Can you work these out from the model? Positions are in its coordinate system, mm. Coordinates: 2 decimals unless noted, no trailing zeros. Loops run counter-clockwise (first coordinate to the right, second up) from the corner with the lowest first, then second, coordinate; pieces in that order, holes last. Notation, with made-up numbers: M 55.5,26 L 65.5,26 A13 ccw 65.5,51 Z; hole C 2.25,-30.5 d7. An arc over 180 degrees is marked long. Answer as a JSON object with one key per item and string values. Group by question number.
Item 1: Suppose I cut it at C-C (y = -11). Write out the boundary of the cut face in (x, z).
Item 2: I'm going to push a flat-ended pin straight in: pin 1 Ø2 at (y, z) = (-6, 1) entering from -X. Where does the tip first touch, or does it pass through?
Item 3: Suppose I cut it at A-A (z = 0). Write out the boundary of the cut face in (x, y), then the cut area to 3 significant figures.
Item 4: Suppose I cut it at B-B (y = 2.75). Write out the boundary of the cut face in (x, z), then the cut area to 3 significant figures.
Item 5: If I drill on line 1 (X direction, y = -0.25, z = 0); line 2 (X direction, y = -11.25, z = 0.75); line 3 (Y direction, x = -1.25, z = -3), over which ranges is the centre line in solid material (lowest first)?
Item 6: We'd pull the mould along X, two halves only. Please class faces 1 (the flat face through (2, 3.781, 0)), 2 (the cylindrical face through (-0.1, -5.3, -2.5)), 3 (the flat face through (0.37, 3.02, 0.06)), 4 (the flat face through (-0.38, 3.04, 0.06)): +X half, -X half, draft (parallel to the pull), parting line (faces both ways), or undercut.
```python
from build123d import *

# Parameters (mm, degrees)
EXTRUDE1_DEPTH = 5


with BuildPart() as part:
    # Sketch1 → Revolve1 (revolve)
    with BuildSketch(Plane.XY, mode=Mode.PRIVATE) as revolve1_sk:
        Polygon((0, 3.780981067), (4.5, 3.780981067), (2.5, 1.780981067), (2.5, -12.219018933), (0, -12.219018933), align=None)
    revolve(revolve1_sk.sketch.rotate(Axis((0, 84.539156627, 0), (0, -1, 0)), 90), axis=Axis((0, 84.539156627, 0), (0, -1, 0)))

    # Sketch2 → Extrude1 (cut, symmetric)
    with BuildSketch(Plane.XY):
        Polygon((-0.75, 3.780981067), (0, 2.280981067), (0.75, 3.780981067), align=None)
    extrude(amount=EXTRUDE1_DEPTH, both=True, mode=Mode.SUBTRACT)


solid = part.part
```
From the geometry:
{
 "1": {"outline": "C 0,0 d5"},
 "2": {"pin 1": "x = -2.5"},
 "3": {"outline": "M -4.5,3.78 L -2.5,1.78 L -2.5,-12.22 L 2.5,-12.22 L 2.5,1.78 L 4.5,3.78 L 0.75,3.78 L 0,2.28 L -0.75,3.78 Z", "area": "82.9 mm2"},
 "4": {"outline": "M -0.23,-3.46 L -0.23,3.46 A3.47 ccw Z; M 0.23,-3.46 A3.47 ccw 0.23,3.46 Z", "area": "34.6 mm2"},
 "5": {"line 1": "-2.5 to 2.5", "line 2": "-2.38 to 2.38", "line 3": "2.53 to 3.78"},
 "6": {"face 1": "draft", "face 2": "parting line", "face 3": "undercut", "face 4": "undercut"}
}
